The listing builds one solid part. Answer for the finished solid, in the listing's coordinates (mm). A direction names the side the tool comes from. Round coordinates to 2 decimals unless told otherwise and drop trailing zeros. Write each loop counter-clockwise with the first axis right and the second up, starting at its lowest first coordinate (ties: lowest second). Pieces come first, ordered by that corner, then holes.
Item 1: Find the intervals of material crossed by probe 1 along X at (y, z) = (9, 5.5); probe 2 along X at (y, z) = (11, 1.5); probe 3 along X at (y, z) = (25, 2.75), in increasing order.
Item 2: For a pull along Y with two mould halves and no side action, classify faces 1 (the face through (12.489, 2.413, 7.395)), 2 (the face through (54, 2, 7)), 3 (the face through (0, 1, 7)), 4 (the face through (49, 0, 7)) as +Y half, -Y half, draft (parallel to the pull), parting line (faces both ways), or undercut.
Item 3: Find section D-D on y = 5.5. Give the vertices of the cut face in (x, z).
Item 4: Find section B-B on y = 23. Give the vertices of the cut face in (x, z), then the cut area to 3 significant figures.
Item 5: A tool of negligible diameter and unlimited length cuts with its end or side. For faces 5 (the face through (26.096, 25.2, 7.395)), 6 (the face through (70.425, 23.348, 7.395)), 7 (the face through (9, 2, 7)), from which of +Z, -Z, +X, -X, +Y, -Y can it reach the whole face along a straight path? Write none if from no direction.
Item 6: Find section C-C on z = 2.5. Give the vertices of the cut face in (x, y), then the cut area to 3 significant figures.
Item 7: Each of these flat-tipped pins is pushed along its axis until it touches: pin 1 (4 mm diameter, centred on x = 14.5, z = 11, fed in from -Y); pin 2 (3 mm diameter, centred on x = 80.5, z = 9, fed in from +Y); pin 3 (7.5 mm diameter, centred on x = 66, z = 8.5, fed in from +Y); pin 4 (1 mm diameter, centred on y = 31.5, z = 3, fed in from +X). Where does it stop, or does it pass through?
Item 8: Find section A-A on x = 48.5. Give the vertices of the cut face in (y, z), then the cut area to 3 significant figures.
```python
from build123d import *

# Parameters (mm, degrees)
BOSS_EXTRUDE1_DEPTH = 15


with BuildPart() as part:
    # Sketch1 → Boss-Extrude1 (new body)
    with BuildSketch(Plane.XY):
        with BuildLine():
            Line((0, 0), (100, 0))
            Line((100, 0), (100, 2))
            Line((100, 2), (40.011106999, 45.301270189))
            Line((40.011106999, 45.301270189), (38.279056191, 46.301270189))
            Line((38.279056191, 46.301270189), (13.567731326, 3.5))
            ThreePointArc((13.567731326, 3.5), (12.469655115, 2.401923789), (10.969655115, 2))
            Line((10.969655115, 2), (7.505553499, 2))
            ThreePointArc((7.505553499, 2), (4.907477288, 3.5), (4.907477288, 6.5))
            Line((4.907477288, 6.5), (10.732050808, 16.588457268))
            Line((10.732050808, 16.588457268), (9, 17.588457268))
            Line((9, 17.588457268), (0, 2))
            Line((0, 2), (0, 0))
        make_face()
        with BuildLine():
            Line((87.30088378, 2), (20.207259422, 2))
            ThreePointArc((20.207259422, 2), (17.60918321, 3.5), (17.60918321, 6.5))
            Line((17.60918321, 6.5), (37.345181053, 40.683751002))
            ThreePointArc((37.345181053, 40.683751002), (39.31497907, 42.117224457), (41.699088187, 41.616251315))
            Line((41.699088187, 41.616251315), (89.056714702, 7.432500313))
            ThreePointArc((89.056714702, 7.432500313), (90.15548541, 4.07736815), (87.30088378, 2))
        make_face(mode=Mode.SUBTRACT)
    extrude(amount=BOSS_EXTRUDE1_DEPTH)


solid = part.part
```
Check values:
1. probe 1: x = 4.04 to 6.35, 16.74 to 19.05, 86.89 to 90.3
1. probe 2: x = 5.2 to 7.51, 17.9 to 20.21, 84.11 to 87.53
1. probe 3: x = 25.98 to 28.29, 64.72 to 68.14
2. face 1: +Y half
2. face 2: undercut
2. face 3: draft
2. face 4: -Y half
3. outline: (2.02, 0) - (4.55, 0) - (4.55, 15) - (2.02, 15) - close; (14.72, 0) - (17.25, 0) - (17.25, 15) - (14.72, 15) - close; (90.26, 0) - (95.15, 0) - (95.15, 15) - (90.26, 15) - close
4. outline: (24.83, 0) - (27.14, 0) - (27.14, 15) - (24.83, 15) - close; (67.49, 0) - (70.91, 0) - (70.91, 15) - (67.49, 15) - close
4. area: 85.9 mm2
5. face 5: +Z, -Z, +Y
5. face 6: +Z, -Z, +X, +Y
5. face 7: +Z, -Z
6. outline: (0, 0) - (100, 0) - (100, 2) - (40.01, 45.3) - (38.28, 46.3) - (13.57, 3.5) arc R3 cw to (10.97, 2) - (7.51, 2) arc R3 cw to (4.91, 6.5) - (10.73, 16.59) - (9, 17.59) - (0, 2) - close; hole (17.61, 6.5) arc R3 ccw to (20.21, 2) - (87.3, 2) arc R3 ccw to (89.06, 7.43) - (41.7, 41.62) arc R3 ccw to (37.35, 40.68) - close
6. area: 513 mm2
7. pin 1: stops at y = 0
7. pin 2: stops at y = 17.16
7. pin 3: stops at y = 29.25
7. pin 4: stops at x = 59.82
8. outline: (0, 0) - (2, 0) - (2, 15) - (0, 15) - close; (36.71, 0) - (39.17, 0) - (39.17, 15) - (36.71, 15) - close
8. area: 67.0 mm2
